The listing builds one solid part. Answer for the finished solid, in the listing's coordinates (mm). Coordinates: 2 decimals unless noted, no trailing zeros. Loops run counter-clockwise (first coordinate to the right, second up) from the corner with the lowest first, then second, coordinate; pieces in that order, holes last. Notation, with made-up numbers: M 74.25,44.5 L 117.25,44.5 A11 ccw 117.25,64.5 Z; hole C 77,-13 d8. An arc over 180 degrees is marked long. Return JSON: item names as keys, results as strings. Group by question number.
1. Straight lines are drawn through the part: L1, parallel to Y at x = 5, z = -2.5; L2, parallel to Y at x = -14.5, z = -3; L3, parallel to X at y = 2, z = 19. For each, find the intervals that lie inside material, in ascending order. Write a range as from..to.
2. Section B-B (x = 2) is taken. Write down the section's boundary in (y, z).
3. Section A-A (z = 9) is taken. Write down the section's boundary in (x, y).
4. Given P1, Ø5, axis at x = 1, y = 7, coming from the -Z side; P2, Ø0.8, axis at x = 10.5, y = 4, coming from the +Z side, each flat-ended and moving along its own axis, determine where each tip first touches the part or whether it passes through.
5. Section C-C (y = 6.5) is taken. Write down the section's boundary in (x, z), then the cut area to 3 significant figures.
6. Section D-D (x = -10.5) is taken. Write down the section's boundary in (y, z), then the cut area to 3 significant figures.
```python
from build123d import *

# Parameters (mm, degrees)
SKETCH1_W           = 41.1
SKETCH1_H           = 41.1
BOSS_EXTRUDE1_DEPTH = 12.5
SKETCH2_W           = 14.5
SKETCH2_H           = 1.6
SKETCH2_W_2         = 6.5
SKETCH2_H_2         = 1.1
CUT_EXTRUDE1_DEPTH  = 30
SKETCH3_W           = 8.369195437
SKETCH3_H           = 2.894608948
BOSS_EXTRUDE2_DEPTH = 3


with BuildPart() as part:
    # Sketch1 → Boss-Extrude1 (new body)
    with BuildSketch(Plane(origin=(0, 0, 0), x_dir=(1, 0, 0), z_dir=(0, 1, 0))):
        Rectangle(SKETCH1_W, SKETCH1_H)
    extrude(amount=BOSS_EXTRUDE1_DEPTH)

    # Sketch2 → Cut-Extrude1 (cut)
    with BuildSketch(Plane.XY.offset(20.55)):
        with Locations((7.3, 6.7)):
            Rectangle(SKETCH2_W, SKETCH2_H)
        with Locations((7.3, 3.9)):
            Rectangle(SKETCH2_W, SKETCH2_H)
        with Locations((-15, 4.55)):
            Rectangle(SKETCH2_W_2, SKETCH2_H_2)
        with Locations((-15, 2.35)):
            Rectangle(SKETCH2_W_2, SKETCH2_H_2)
    extrude(amount=-CUT_EXTRUDE1_DEPTH, mode=Mode.SUBTRACT)

    # Sketch3 → Boss-Extrude2 (add)
    with BuildSketch(Plane(origin=(0, 0, -20.55), x_dir=(-1, 0, 0), z_dir=(0, 0, -1))):
        with Locations((-14.504507882, 6.024959093)):
            Rectangle(SKETCH3_W, SKETCH3_H)
    extrude(amount=BOSS_EXTRUDE2_DEPTH)


solid = part.part
```
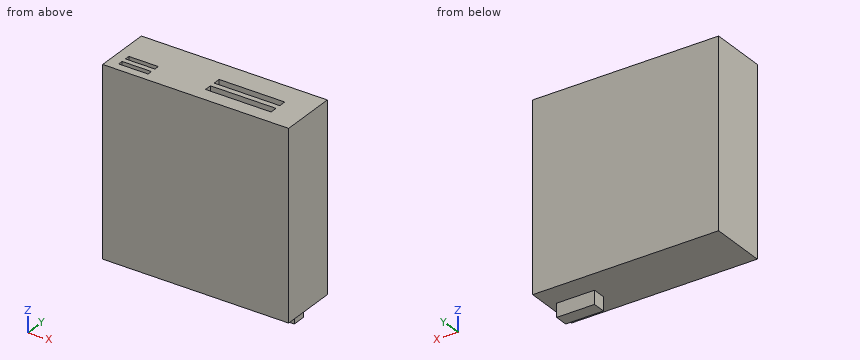
Worked out:
{
 "1": {"L1": "0..3.1, 4.7..5.9, 7.5..12.5", "L2": "0..1.8, 2.9..4, 5.1..12.5", "L3": "-20.55..-18.25, -11.75..20.55"},
 "2": {"outline": "M 0,-20.55 L 12.5,-20.55 L 12.5,20.55 L 7.5,20.55 L 7.5,-9.45 L 5.9,-9.45 L 5.9,20.55 L 4.7,20.55 L 4.7,-9.45 L 3.1,-9.45 L 3.1,20.55 L 0,20.55 Z"},
 "3": {"outline": "M -20.55,0 L 20.55,0 L 20.55,12.5 L -20.55,12.5 Z; hole M -18.25,1.8 L -11.75,1.8 L -11.75,2.9 L -18.25,2.9 Z; hole M -18.25,4 L -11.75,4 L -11.75,5.1 L -18.25,5.1 Z; hole M 0.05,3.1 L 14.55,3.1 L 14.55,4.7 L 0.05,4.7 Z; hole M 0.05,5.9 L 14.55,5.9 L 14.55,7.5 L 0.05,7.5 Z"},
 "4": {"P1": "z = -20.55", "P2": "z = -9.45"},
 "5": {"outline": "M -20.55,-20.55 L 10.32,-20.55 L 10.32,-23.55 L 18.69,-23.55 L 18.69,-20.55 L 20.55,-20.55 L 20.55,20.55 L 14.55,20.55 L 14.55,-9.45 L 0.05,-9.45 L 0.05,20.55 L -20.55,20.55 Z", "area": "1,280 mm^2"},
 "6": {"outline": "M 0,-20.55 L 12.5,-20.55 L 12.5,20.55 L 0,20.55 Z", "area": "514 mm^2"}
}
